from build123d import *

# Parameters (mm, degrees)
SKETCH1_W           = 105
SKETCH1_H           = 10
SKETCH1_R           = 1.5
BOSS_EXTRUDE1_DEPTH = 3
SKETCH2_W           = 10.5
SKETCH2_H           = 3
CUT_EXTRUDE1_DEPTH  = 53.82281704


with BuildPart() as part:
    # Sketch1 → Boss-Extrude1 (new body)
    with BuildSketch(Plane(origin=(0, 0, 0), x_dir=(1, 0, 0), z_dir=(0, 1, 0))):
        Rectangle(SKETCH1_W, SKETCH1_H)
        with Locations(Location((0, 0, 0), (0, 0, 270))):
            Circle(SKETCH1_R, mode=Mode.SUBTRACT)
    extrude(amount=BOSS_EXTRUDE1_DEPTH)

    # Sketch2 → Cut-Extrude1 (cut, through all)
    with BuildSketch(Plane(origin=(0, 3, 0), x_dir=(1, 0, 0), z_dir=(0, 1, 0))):
        with Locations((-47.25, -3.5)):
            Rectangle(SKETCH2_W, SKETCH2_H)
    cut_extrude1 = extrude(amount=-CUT_EXTRUDE1_DEPTH, mode=Mode.SUBTRACT)

    # Mirror2: Cut-Extrude1 across plane
    add(cut_extrude1.mirror(Plane(origin=(0, 0, 0), x_dir=(0, 0, 1), z_dir=(1, 0, 0))), mode=Mode.SUBTRACT)


solid = part.part
For this review, take the finished solid that the model builds, in its own axes (mm). A direction names the side the tool comes from. Round coordinates to 2 decimals unless told otherwise and drop trailing zeros. Write each loop counter-clockwise with the first axis right and the second up, starting at its lowest first coordinate (ties: lowest second). Pieces come first, ordered by that corner, then holes. Notation, with made-up numbers: M 67,25.25 L 83,25.25 A25 cw 83,55.25 Z; hole C -39.75,63 d8. An arc over 180 degrees is marked long. Write item = value, one per line. Start each with the question number.
(1) For line 1 along X through (y, z) = (2.35, 0); line 2 along X through (y, z) = (0.55, 2.5); line 3 along X through (y, z) = (0.95, 0.5), list the stretches that pass through material, from the lowest coordinate up.
(2) We need section A-A (z = 0). Give the boundary of the cut face in (x, y), then the cut area to 3 significant figures.
(3) We need section C-C (y = 1.45). Give the boundary of the cut face in (x, z), then the cut area to 3 significant figures.
(4) For faces 5 (the face through (47, 2, 2)), 6 (the face through (-47, 2, 2)), 7 (the face through (-1, 1, 5)), list the 3-axis set-ups (+Z, -Z, +X, -X, +Y, -Y) from which the entire face can be reached by the end or side of a thin tool; tool diameter is ignored.
(5) The part is to be moulded in two halves that separate along X. For faces 1 (the face through (-42, 2, 4)), 2 (the face through (-1, 1, -5)), 3 (the face through (42, 2, 4)), 4 (the face through (0.45, 1.48, 1.43)), say which applies: +X half, -X half, draft (parallel to the pull), parting line (faces both ways), or undercut.
(6) We need section B-B (x = 0). Give the boundary of the cut face in (y, z), then the cut area to 3 significant figures.
(7) Clearance check with a flat-ended pin moving along its axis: pin 1 Ø0.9 at (x, y) = (-49, 2) entering from +Z. State where the tip first meets the part, or that it passes through.
Results found:
q1.line_1 = -52.5 to -1.5, 1.5 to 52.5
q1.line_2 = -42 to 42
q1.line_3 = -52.5 to -1.41, 1.41 to 52.5
q2.outline = M -52.5,0 L -1.5,0 L -1.5,3 L -52.5,3 Z; M 1.5,0 L 52.5,0 L 52.5,3 L 1.5,3 Z
q2.area = 306 mm²
q3.outline = M -52.5,-5 L 52.5,-5 L 52.5,2 L 42,2 L 42,5 L -42,5 L -42,2 L -52.5,2 Z; hole C 0,0 d3
q3.area = 980 mm²
q4.face_5 = +Z, +X, +Y, -Y
q4.face_6 = +Z, -X, +Y, -Y
q4.face_7 = +Z, +X, -X, +Y, -Y
q5.face_1 = -X half
q5.face_2 = draft
q5.face_3 = +X half
q5.face_4 = undercut
q6.outline = M 0,-5 L 3,-5 L 3,-1.5 L 0,-1.5 Z; M 0,1.5 L 3,1.5 L 3,5 L 0,5 Z
q6.area = 21.0 mm²
q7.pin_1 = 2
